CAD build for the part. Positions are in the model's coordinates, mm. A direction names the side the tool comes from. Coordinates: 2 decimals unless noted, no trailing zeros. Order: outer loops, then holes, each group sorted by start corner. A loop starts at its lowest first (then second) coordinate and runs counter-clockwise, first axis right, second up. Notation, with made-up numbers: (54, -29.75) -> (96, -29.75) arc R8 cw to (96, -18.75) -> close; hole circle Ø4 at (-29.75, 52). An arc over 180 degrees is marked (long way). Use one line per item in the form item = value. Start each with the question number.
from build123d import *

# Parameters (mm, degrees)
SKETCH_W      = 50
SKETCH_H      = 50
PAD_DEPTH     = 3
SKETCH001_W   = 50
SKETCH001_H   = 50
SKETCH001_W_2 = 44
SKETCH001_H_2 = 44
PAD001_DEPTH  = 27.7
SKETCH002_R   = 2.5
PAD002_DEPTH  = 27.7
SKETCH003_R   = 1.05
HOLE_DEPTH    = 25
HOLE_TIPS_R   = 1.05


with BuildPart() as part:
    # Sketch → Pad (new body)
    with BuildSketch(Plane.XY):
        Rectangle(SKETCH_W, SKETCH_H)
    extrude(amount=PAD_DEPTH)

    # Sketch001 (on Face6 of Pad) → Pad001 (join)
    with BuildSketch(Plane.XY.offset(3)):
        Rectangle(SKETCH001_W, SKETCH001_H)
        Rectangle(SKETCH001_W_2, SKETCH001_H_2, mode=Mode.SUBTRACT)
    extrude(amount=PAD001_DEPTH)

    # Sketch002 (on Face15 of Pad001) → Pad002 (join)
    with BuildSketch(Plane.XY.offset(3)):
        with Locations((-17, 17)):
            Circle(SKETCH002_R)
        with Locations((17, 17)):
            Circle(SKETCH002_R)
        with Locations((17, -17)):
            Circle(SKETCH002_R)
        with Locations((-17, -17)):
            Circle(SKETCH002_R)
    extrude(amount=PAD002_DEPTH)

    # Sketch003 (on Face22 of Pad002) → Hole (cut)
    with BuildSketch(Plane.XY.offset(30.7)):
        with Locations((-17, 17)):
            Circle(SKETCH003_R)
        with Locations((17, 17)):
            Circle(SKETCH003_R)
        with Locations((-17, -17)):
            Circle(SKETCH003_R)
        with Locations((17, -17)):
            Circle(SKETCH003_R)
    extrude(amount=-HOLE_DEPTH, mode=Mode.SUBTRACT)

    # Hole tips → Hole tip 1 section 0
    with BuildSketch(Plane.XY.offset(5.7), mode=Mode.PRIVATE) as hole_tip_1_s0:
        with Locations((-17, 17)):
            Circle(HOLE_TIPS_R)
    loft([hole_tip_1_s0.sketch, Vertex(-17, 17, 5.069096)], mode=Mode.SUBTRACT)

    # Hole tips → Hole tip 2 section 0
    with BuildSketch(Plane.XY.offset(5.7), mode=Mode.PRIVATE) as hole_tip_2_s0:
        with Locations((17, 17)):
            Circle(HOLE_TIPS_R)
    loft([hole_tip_2_s0.sketch, Vertex(17, 17, 5.069096)], mode=Mode.SUBTRACT)

    # Hole tips → Hole tip 3 section 0
    with BuildSketch(Plane.XY.offset(5.7), mode=Mode.PRIVATE) as hole_tip_3_s0:
        with Locations((-17, -17)):
            Circle(HOLE_TIPS_R)
    loft([hole_tip_3_s0.sketch, Vertex(-17, -17, 5.069096)], mode=Mode.SUBTRACT)

    # Hole tips → Hole tip 4 section 0
    with BuildSketch(Plane.XY.offset(5.7), mode=Mode.PRIVATE) as hole_tip_4_s0:
        with Locations((17, -17)):
            Circle(HOLE_TIPS_R)
    loft([hole_tip_4_s0.sketch, Vertex(17, -17, 5.069096)], mode=Mode.SUBTRACT)


solid = part.part
1) Cut at A-A on z = 12.5. Count the separate pieces of the cut face and the enclosed holes in it, then the cut area to 3 significant figures.
2) Drop a flat-ended pin along its axis: P1, Ø3, axis at x = -13, y = 2, coming from the +Z side. Give the stop position or say it passes through.
3) Two-plate mould, pull along X, no slides. Class faces 3 (the face through (0, 0, 0)), 4 (the face through (25, 0, 15)), 5 (the face through (-22, 0, 17)): released by +X, released by -X, zero draft, split by the parting line, or undercut.
4) Probe L1, parallel to Y at x = 17, z = 23; L2, parallel to Y at x = 3.5, z = 9. List the from-to ranges inside material, lowest first.
5) Cut at B-B on x = -4. Give the cut face in (y, z), then the cut area to 3 significant figures.
6) 3-axis set-ups, long thin cutter, end or side, ignore diameter. For faces 1 (the face through (0, 22, 17)), 2 (the face through (-25, 0, 15)): which of +Z, -Z, +X, -X, +Y, -Y reach the whole face in a straight line?
Values follow:
q1.separate_pieces = 5
q1.enclosed_holes = 5
q1.area = 629 mm^2
q2.P1 = 3
q3.face_3 = zero draft
q3.face_4 = released by +X
q3.face_5 = undercut
q4.L1 = -25 to -22, -19.5 to -18.05, -15.95 to -14.5, 14.5 to 15.95, 18.05 to 19.5, 22 to 25
q4.L2 = -25 to -22, 22 to 25
q5.outline = (-25, 0) -> (25, 0) -> (25, 30.7) -> (22, 30.7) -> (22, 3) -> (-22, 3) -> (-22, 30.7) -> (-25, 30.7) -> close
q5.area = 316 mm^2
q6.face_1 = +Z
q6.face_2 = +Z, -Z, -X, +Y, -Y
